Geometry: final body of the model. Coordinates: model frame, mm. Face numbers are marked on the shaded views. A direction names the side the tool comes from. Round coordinates to 2 decimals unless told otherwise and drop trailing zeros. Write each loop counter-clockwise with the first axis right and the second up, starting at its lowest first coordinate (ties: lowest second). Pieces come first, ordered by that corner, then holes. Notation, with made-up numbers: (24, 6) - (46, 6) arc R21 ccw to (46, 42) - close; hole circle Ø1 at (12.25, 32.25). An arc over 180 degrees is marked (long way). Use a Markdown table: item, result. Add a question column.
```python
from build123d import *

# Parameters (mm, degrees)
F2_DEPTH = 7
F3_R     = 11.5
F4_DEPTH = 25.4


with BuildPart() as f2:
    # F1 (on Top) → F2 (new body)
    with BuildSketch(Plane.XY):
        with BuildLine():
            ThreePointArc((-10.747828, 17.888175), (-10.389928, 9.784178), (-17.137527, 14.286707))
            Line((-17.137527, 14.286707), (-44.084065, 13.019221))
            Line((-44.084065, 13.019221), (-21.436056, -4.069164))
            ThreePointArc((-21.436056, -4.069164), (-12.818896, -4.786043), (-19.344879, -10.458865))
            Line((-19.344879, -10.458865), (-27.523644, -37.316266))
            Line((-27.523644, -37.316266), (-4.706655, -21.727975))
            ThreePointArc((-4.706655, -21.727975), (-0.92379, -14.017584), (2.612456, -21.844152))
            Line((2.612456, -21.844152), (25.1483, -38.559195))
            Line((25.1483, -38.559195), (18.180093, -11.62063))
            ThreePointArc((18.180093, -11.62063), (12.489564, -5.416127), (20.735973, -3.720635))
            Line((20.735973, -3.720635), (43.389283, 13.194266))
            Line((43.389283, 13.194266), (15.262693, 15.336566))
            ThreePointArc((15.262693, 15.336566), (8.257426, 10.799074), (9.541669, 19.046092))
            Line((9.541669, 19.046092), (-0.92379, 43.835886))
            Line((-0.92379, 43.835886), (-10.747828, 17.888175))
        make_face()
    extrude(amount=-F2_DEPTH)

    # F3 (on face) → F4 (cut)
    with BuildSketch(Plane.XY):
        Circle(F3_R)
    extrude(amount=-F4_DEPTH, mode=Mode.SUBTRACT)


solid = f2.part
```
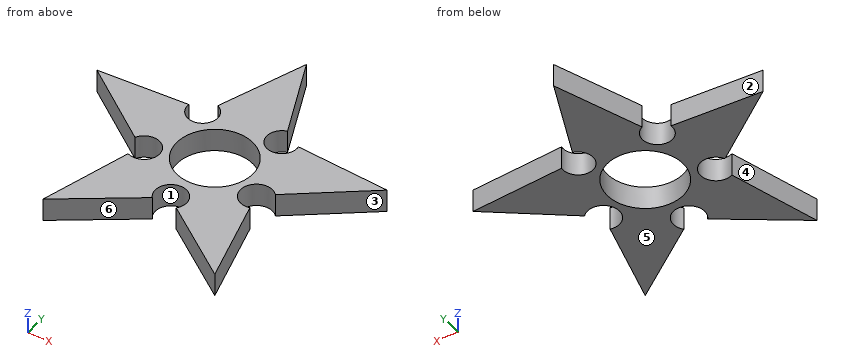
1) Pin query (flat end, axial travel): P1, Ø4, axis at x = -21.5, z = -2.5, coming from the -Y side; P2, Ø4, axis at y = -26.5, z = -1.5, coming from the -X side; P3, Ø4, axis at y = 34, z = -4.5, coming from the +X side. Return the tip coordinate at first contact, or that it passes through.
2) Section C-C, the plane x = -3. Return the cut outline in (y, z).
3) Material intervals for L1, parallel to X at y = -23.5, z = -1; L2, parallel to X at y = -10, z = -4.5; L3, parallel to X at y = 10.5, z = -2.75, sorted ascending. Write a range as from..to.
4) Section A-A, the plane z = -4.5. Return the cut outline in (x, y), then the cut area to 3 significant figures.
5) Section B-B, the plane y = -8. Return the cut outline in (x, z).
6) Draft query along X for the marked faces 1, 2 and 3. Return one class per face: released by +X, released by -X, zero draft, split by the parting line, or undercut.
7) Section D-D, the plane y = 38. Return the cut outline in (x, z), then the cut area to 3 significant figures.
8) Set-up query: the marked faces 4, 5 and 6. Return all of +Z, -Z, +X, -X, +Y, -Y with unobstructed straight access to the full face (end or side cutting, diameter ignored); none if empty.
Output values:
| question | item | result |
|---|---|---|
| 1 | P1 | stops at y = -34.57 |
| 1 | P2 | stops at x = -24.84 |
| 1 | P3 | stops at x = 4.07 |
| 2 | outline | (-14.46, -7) - (-11.1, -7) - (-11.1, 0) - (-14.46, 0) - close; (11.1, -7) - (38.35, -7) - (38.35, 0) - (11.1, 0) - close |
| 3 | L1 | x = -23.32..-7.3, 4.84..21.25 |
| 3 | L2 | x = -14.46..-5.68, 5.68..13.37 |
| 3 | L3 | x = -40.75..-15.81, -9.44..-4.69, 4.69..8.79, 12.69..39.78 |
| 4 | outline | (-44.08, 13.02) - (-21.44, -4.07) arc R4.69 cw (long way) to (-19.34, -10.46) - (-27.52, -37.32) - (-4.71, -21.73) arc R4.75 cw (long way) to (2.61, -21.84) - (25.15, -38.56) - (18.18, -11.62) arc R4.84 cw (long way) to (20.74, -3.72) - (43.39, 13.19) - (15.26, 15.34) arc R4.57 cw (long way) to (9.54, 19.05) - (-0.92, 43.84) - (-10.75, 17.89) arc R4.55 cw (long way) to (-17.14, 14.29) - close; hole circle Ø23 at (0, 0) |
| 4 | area | 1,860 mm^2 |
| 5 | outline | (-12.93, -7) - (-8.26, -7) - (-8.26, 0) - (-12.93, 0) - close; (8.26, -7) - (12.38, -7) - (12.38, 0) - (8.26, 0) - close |
| 6 | face 1 | undercut |
| 6 | face 2 | released by -X |
| 6 | face 3 | released by +X |
| 7 | outline | (-3.13, -7) - (1.54, -7) - (1.54, 0) - (-3.13, 0) - close |
| 7 | area | 32.7 mm^2 |
| 8 | face 4 | +Z, -Z, -X |
| 8 | face 5 | -Z, +X, -X, +Y, -Y |
| 8 | face 6 | +Z, -Z, -Y |
